Can you work these out from the model? Positions are in its coordinate system, mm. A direction names the side the tool comes from. Coordinates: 2 decimals unless noted, no trailing zeros. Order: outer loops, then holes, each group sorted by start corner. A loop starts at its lowest first (then second) coordinate and runs counter-clockwise, first axis right, second up. Notation, with made-up numbers: (-11, 85) -> (45, 85) arc R31 ccw to (45, 114) -> close; hole circle Ø1 at (67.5, 21.5). An arc over 180 degrees is marked (long way). Answer as CSV lines item,"result".
from build123d import *

# Parameters (mm, degrees)
F1_DEPTH       = 508
F2_W           = 546.1
F2_H           = 203.2
F3_DEPTH       = 635
F6_DEPTH       = 508
F8_D           = 86.36
F8_CSINK_D     = 200.66
F8_CSINK_ANGLE = 90


with BuildPart() as f1:
    # F0 (on Front) → F1 (new body)
    with BuildSketch(Plane.XZ):
        Polygon((0, 279.4), (0, 0), (254, 0), (254, 237.349615), (129.794, 279.4), align=None)
    extrude(amount=F1_DEPTH)

    # F2 (on Front) → F3 (join)
    with BuildSketch(Plane.XZ):
        with Locations((527.05, 101.6)):
            Rectangle(F2_W, F2_H)
    extrude(amount=F3_DEPTH)

    # F5 (on face) → F6 (join)
    with BuildSketch(Plane(origin=(0, 0, 0), x_dir=(-1, 0, 0), z_dir=(0, 1, 0))):
        Polygon((0, 279.4), (-129.794, 279.4), (-254, 237.349615), (-254, 203.2), (-254, 0), (0, 0), align=None)
        Polygon((-1054.1, 279.4), (-1054.1, 0), (-800.1, 0), (-800.1, 203.2), (-800.1, 237.349615), (-924.306, 279.4), align=None)
    extrude(amount=-F6_DEPTH)

    # F8 (through all)
    with Locations(Plane.XY.offset(203.2)):
        with Locations((660.4, -508), (393.7, -508), (393.7, -127), (660.4, -127)):
            CounterSinkHole(F8_D / 2, F8_CSINK_D / 2, counter_sink_angle=F8_CSINK_ANGLE)


solid = f1.part
Q1. Imagine slicing it at B-B (z = 190.5). List the corners of the cut face in (x, y) for me.
Solution:
outline,"(0, -508) -> (254, -508) -> (254, -635) -> (800.1, -635) -> (800.1, -508) -> (1054.1, -508) -> (1054.1, 0) -> (0, 0) -> close; hole circle Ø175.26 at (393.7, -508); hole circle Ø175.26 at (393.7, -127); hole circle Ø175.26 at (660.4, -508); hole circle Ø175.26 at (660.4, -127)"
Q2. We'd pull the mould along Y, two halves only. Please class faces 5 (the cylindrical face through (637.19, -90.59, 72)), 6 (the flat face through (523, -635, 103)), 7 (the flat face through (0, -250, 142)): pulls with the +Y half, pulls with the -Y half, needs draft (parallel to the pull), parting line crosses it, or undercut.
Solution:
face 5,"undercut"
face 6,"pulls with the -Y half"
face 7,"needs draft"
Q3. If I drill on line 1 (Y direction, x = 393.7, z = 77.5); line 2 (X direction, y = -127, z = 94); line 3 (X direction, y = -95, z = 20), over which ranges is the centre line in solid material (lowest first)?
Solution:
line 1,"-635 to -551.18, -464.82 to -170.18, -83.82 to 0"
line 2,"0 to 350.52, 436.88 to 617.22, 703.58 to 1054.1"
line 3,"0 to 364.71, 422.69 to 631.41, 689.39 to 1054.1"
Q4. Imagine slicing it at D-D (x = 538.5). List the corners of the cut face in (y, z) for me.
Solution:
outline,"(-635, 0) -> (0, 0) -> (0, 203.2) -> (-635, 203.2) -> close"
Q5. Imagine slicing it at A-A (x = 393.7). List the corners of the cut face in (y, z) for me, and give its area (3 significant figures).
Solution:
outline,"(-635, 0) -> (-551.18, 0) -> (-551.18, 146.05) -> (-608.33, 203.2) -> (-635, 203.2) -> close; (-464.82, 0) -> (-170.18, 0) -> (-170.18, 146.05) -> (-227.33, 203.2) -> (-407.67, 203.2) -> (-464.82, 146.05) -> close; (-83.82, 0) -> (0, 0) -> (0, 203.2) -> (-26.67, 203.2) -> (-83.82, 146.05) -> close"
area,"87,400 mm2"
Q6. Which directions (+Z, -Z, +X, -X, +Y, -Y) give clear straight access to the entire face, cutting with the end or side of a thin tool? Please do faces 1 (the flat face through (929, -508, 142)), 2 (the flat face through (254, -571, 100)), 3 (the cylindrical face through (425.53, -478.82, 72)), 4 (the flat face through (193, -250, 258)).
Solution:
face 1,"+Z, -Z, +X, -Y"
face 2,"+Z, -Z, -X, -Y"
face 3,"+Z, -Z"
face 4,"+Z, +Y, -Y"
Q7. Imagine slicing it at C-C (y = -382). List the corners of the cut face in (x, z) for me.
Solution:
outline,"(0, 0) -> (1054.1, 0) -> (1054.1, 279.4) -> (924.31, 279.4) -> (800.1, 237.35) -> (800.1, 203.2) -> (254, 203.2) -> (254, 237.35) -> (129.79, 279.4) -> (0, 279.4) -> close"
Q8. For P1, Ø1.5, axis at x = 913, y = -147.5, coming from the +Z side; P2, Ø10, axis at y = -542.5, z = 133.5, coming from the -X side, each with a flat end and sliding along its axis, tell me the tip position at first contact or that it passes through.
Solution:
P1,"z = 275.83"
P2,"x = 254"
